Check sheet for the modelled part. Datum: model origin and axes. Units: mm. Coordinates: 2 decimals unless noted, no trailing zeros. Write each loop counter-clockwise with the first axis right and the second up, starting at its lowest first coordinate (ties: lowest second). Pieces come first, ordered by that corner, then holes. Notation, with made-up numbers: M 31,24.5 L 46,24.5 A25 cw 46,54.5 Z; hole C 3.25,24.5 d3. An arc over 180 degrees is marked long. Answer as CSV lines item,"result".
Autodesk Inventor part; units mm, degrees
ref_plane "YZ Plane" through (0, 0, 0) normal (1, 0, 0) x (0, 1, 0)
ref_plane "XZ Plane" through (0, 0, 0) normal (0, 1, 0) x (-1, 0, 0)
ref_plane "XY Plane" through (0, 0, 0) normal (0, 0, 1) x (1, 0, 0)
sketch "Sketch1" plane through (0, 0, 0) normal (0, 0, 1) x (1, 0, 0)
  line L0 (0, 0) -> (25, 0)
  arc A0 (7.8015, 18.2899) -> (17.1985, 18.2899) centre (12.5, 20) ccw
  line L1 (18.1364, 18.2945) -> (25, 0)
  line L2 (6.8636, 18.2945) -> (0, 0)
  arc A1 (7.8015, 18.2899) -> (6.8636, 18.2945) centre (7.3317, 18.1189) ccw
  arc A2 (18.1364, 18.2945) -> (17.1985, 18.2899) centre (17.6683, 18.1189) ccw
  dimension "d0" = 5
  dimension "d1" = 20
  dimension "d2" = 25
  dimension "d4" = 20
  dimension "d9" = 0.5
extrude "Extrusion1" add sketch "Sketch1" along normal blind 3.175
equation "\"d5\" = THICKA"
equation "\"THICKA\" = 3.175"
equation "\"THICKB\" = 6.731"
equation "\"THICKC\" = 12.7"
equation "\"MAGDIA\" = 9.5"
equation "\"BALLDIA\" = 12"
properties part number "Air2D_Shaft_Brace"
1) Section check D-D, the plane y = 8.25. Record the boundary of the cut face in (x, z) (3 decimals).
Answer key:
outline,"M 3.095,0 L 21.905,0 L 21.905,3.175 L 3.095,3.175 Z"
2) Section check B-B, the plane z = 2.7. Record the boundary of the cut face in (x, y).
Answer key:
outline,"M 0,0 L 25,0 L 18.14,18.29 A0.5 ccw 17.2,18.29 A5 cw 7.8,18.29 A0.5 ccw 6.86,18.29 Z"
3) Section check A-A, the plane y = 15.75. Record the boundary of the cut face in (x, z) (3 decimals).
Answer key:
outline,"M 5.909,0 L 9.866,0 L 9.866,3.175 L 5.909,3.175 Z; M 15.134,0 L 19.091,0 L 19.091,3.175 L 15.134,3.175 Z"
4) Mould release check, pull along X, two halves, no side actions. Record for faces 1 (the face through (12.6, 15, 1.6)), 2 (the face through (21.52, 9.28, 1.57)), 3 (the face through (12, 0, 2)): pulls with the +X half, pulls with the -X half, needs draft (parallel to the pull), parting line crosses it, or undercut.
Answer key:
face 1,"undercut"
face 2,"pulls with the +X half"
face 3,"needs draft"
5) Depth check by flat-ended pin: P1, Ø10, axis at x = 22.5, y = 4, coming from the -Z side; P2, Ø1.5, axis at x = 15, z = 0.5, coming from the +Y side. Enter the tip coordinate at first touch or a pass-through.
Answer key:
P1,"stops at z = 0"
P2,"stops at y = 16.2"
6) Section check C-C, the plane x = 14.5. Record the boundary of the cut face in (y, z) (3 decimals), plus the area to 3 significant figures.
Answer key:
outline,"M 0,0 L 15.417,0 L 15.417,3.175 L 0,3.175 Z"
area,"49.0 mm2"
7) Thickness scan on line 1 along X through (y, z) = (15.75, 1.3); line 2 along X through (y, z) = (14.5, 2.65); line 3 along Y through (x, z) = (11.75, 1.35). Record the ranges inside material, lowest first.
Answer key:
line 1,"x = 5.91 to 9.87, 15.13 to 19.09"
line 2,"x = 5.44 to 19.56"
line 3,"y = 0 to 15.06"
